Input: part model. Units: mm. Frame: model coordinates. A direction names the side the tool comes from. Round coordinates to 2 decimals unless told otherwise and drop trailing zeros. Write each loop counter-clockwise with the first axis right and the second up, starting at its lowest first coordinate (ties: lowest second). Pieces come first, ordered by that corner, then holes. Notation, with made-up numbers: (60.25, 12.5) -> (80.25, 12.5) arc R11 cw to (80.25, 29.5) -> close; hole circle Ø6 at (-8.75, -35.75). An arc over 180 degrees is marked (long way). Use CSV: the item, a comma, the result in double quotes.
```python
from build123d import *

# Parameters (mm, degrees)
F1_DEPTH = 40
F0_W     = 3
F0_H     = 3
F2_DEPTH = 30
F3_R     = 2
F4_DEPTH = 30
F5_R     = 7.5
F5_R_2   = 5
F6_DEPTH = 5


with BuildPart() as f1:
    # F0 (on Top) → F1 (new body)
    with BuildSketch(Plane.XY):
        with BuildLine():
            ThreePointArc((-4.7696960071, -1.5), (-5, 0), (-4.7696960071, 1.5))
            Line((-4.7696960071, 1.5), (-40, 1.5))
            Line((-40, 1.5), (-40, -1.5))
            Line((-40, -1.5), (-4.7696960071, -1.5))
        make_face()
    extrude(amount=F1_DEPTH)



with BuildPart() as f1b:
    # F0 (on Top) → F1, piece 2 (new body)
    with BuildSketch(Plane.XY):
        with BuildLine():
            ThreePointArc((-1.5, 4.7696960071), (0, 5), (1.5, 4.7696960071))
            Line((1.5, 4.7696960071), (1.5, 40))
            Line((1.5, 40), (-1.5, 40))
            Line((-1.5, 40), (-1.5, 4.7696960071))
        make_face()
    extrude(amount=F1_DEPTH)


with BuildPart() as f1c:
    # F0 (on Top) → F1, piece 3 (new body)
    with BuildSketch(Plane.XY):
        with BuildLine():
            ThreePointArc((4.7696960071, 1.5), (4.9420886291, 0.7587884964), (5, 0))
            ThreePointArc((5, 0), (4.9420886291, -0.7587884964), (4.7696960071, -1.5))
            Line((4.7696960071, -1.5), (40, -1.5))
            Line((40, -1.5), (40, 1.5))
            Line((40, 1.5), (4.7696960071, 1.5))
        make_face()
    extrude(amount=F1_DEPTH)


with BuildPart() as f1d:
    # F0 (on Top) → F1, piece 4 (new body)
    with BuildSketch(Plane.XY):
        with BuildLine():
            Line((1.5, -40), (1.5, -4.7696960071))
            ThreePointArc((1.5, -4.7696960071), (0, -5), (-1.5, -4.7696960071))
            Line((-1.5, -4.7696960071), (-1.5, -40))
            Line((-1.5, -40), (1.5, -40))
        make_face()
    extrude(amount=F1_DEPTH)


with BuildPart() as f1_1:
    add(f1.part)

    add(f1b.part)  # F2 merges F1b

    add(f1c.part)  # F2 merges F1c

    add(f1d.part)  # F2 merges F1d
    # F0 (on Top) → F2 (join)
    with BuildSketch(Plane.XY):
        with BuildLine():
            Line((-1.5, 1.5), (-1.5, 4.7696960071))
            ThreePointArc((-1.5, 4.7696960071), (-3.5355339059, 3.5355339059), (-4.7696960071, 1.5))
            Line((-4.7696960071, 1.5), (-1.5, 1.5))
        make_face()
        with BuildLine():
            Line((1.5, 1.5), (4.7696960071, 1.5))
            ThreePointArc((4.7696960071, 1.5), (3.5355339059, 3.5355339059), (1.5, 4.7696960071))
            Line((1.5, 4.7696960071), (1.5, 1.5))
        make_face()
        with BuildLine():
            ThreePointArc((1.5, -4.7696960071), (3.5355339059, -3.5355339059), (4.7696960071, -1.5))
            Line((4.7696960071, -1.5), (1.5, -1.5))
            Line((1.5, -1.5), (1.5, -4.7696960071))
        make_face()
        with BuildLine():
            ThreePointArc((-4.7696960071, -1.5), (-3.5355339059, -3.5355339059), (-1.5, -4.7696960071))
            Line((-1.5, -4.7696960071), (-1.5, -1.5))
            Line((-1.5, -1.5), (-4.7696960071, -1.5))
        make_face()
        with BuildLine():
            ThreePointArc((4.7696960071, -1.5), (4.9420886291, -0.7587884964), (5, 0))
            ThreePointArc((5, 0), (4.9420886291, 0.7587884964), (4.7696960071, 1.5))
            Line((4.7696960071, 1.5), (1.5, 1.5))
            Line((1.5, 1.5), (1.5, -1.5))
            Line((1.5, -1.5), (4.7696960071, -1.5))
        make_face()
        with BuildLine():
            Line((1.5, 1.5), (1.5, 4.7696960071))
            ThreePointArc((1.5, 4.7696960071), (0, 5), (-1.5, 4.7696960071))
            Line((-1.5, 4.7696960071), (-1.5, 1.5))
            Line((-1.5, 1.5), (1.5, 1.5))
        make_face()
        with BuildLine():
            Line((-1.5, -1.5), (-1.5, 1.5))
            Line((-1.5, 1.5), (-4.7696960071, 1.5))
            ThreePointArc((-4.7696960071, 1.5), (-5, 0), (-4.7696960071, -1.5))
            Line((-4.7696960071, -1.5), (-1.5, -1.5))
        make_face()
        Rectangle(F0_W, F0_H)
        with BuildLine():
            ThreePointArc((-1.5, -4.7696960071), (0, -5), (1.5, -4.7696960071))
            Line((1.5, -4.7696960071), (1.5, -1.5))
            Line((1.5, -1.5), (-1.5, -1.5))
            Line((-1.5, -1.5), (-1.5, -4.7696960071))
        make_face()
    extrude(amount=F2_DEPTH)

    # F3 (on face) → F4 (cut)
    with BuildSketch(Plane.XY.offset(30)):
        Circle(F3_R)
    extrude(amount=-F4_DEPTH, mode=Mode.SUBTRACT)

    # F5 (on face) → F6 (cut)
    with BuildSketch(Plane(origin=(0, 0, 0), x_dir=(1, 0, 0), z_dir=(0, 0, -1))):
        Circle(F5_R)
        Circle(F5_R_2, mode=Mode.SUBTRACT)
    extrude(amount=-F6_DEPTH, mode=Mode.SUBTRACT)


solid = f1_1.part
```
Item 1: Section query A-A on z = 4. Return the cut outline in (x, y).
Worked answers:
outline,"(-40, -1.5) -> (-7.35, -1.5) arc R7.5 cw to (-7.35, 1.5) -> (-40, 1.5) -> close; circle Ø10 at (0, 0); (-1.5, -40) -> (1.5, -40) -> (1.5, -7.35) arc R7.5 cw to (-1.5, -7.35) -> close; (-1.5, 7.35) arc R7.5 cw to (1.5, 7.35) -> (1.5, 40) -> (-1.5, 40) -> close; (7.35, -1.5) -> (40, -1.5) -> (40, 1.5) -> (7.35, 1.5) arc R7.5 cw to start; hole circle Ø4 at (0, 0)"
Item 2: Pull-direction query (Y, two-part tool) for faces 1 (the face through (0, 7.5, 2.5)), 2 (the face through (-22, 1.5, 20)), 3 (the face through (0, -7.5, 2.5)), 4 (the face through (-1.5, -22, 20)); classes: +Y half, -Y half, draft (parallel to the pull), parting line (faces both ways), or undercut.
Worked answers:
face 1,"undercut"
face 2,"+Y half"
face 3,"undercut"
face 4,"draft"
Item 3: First-contact query: pin 1 Ø17.5 at (x, z) = (-17.5, 27.5) entering from +Y; pin 2 Ø10.5 at (x, z) = (-16, 25.5) entering from -Y; pin 3 Ø10.5 at (y, z) = (28, 27.5) entering from -X. Flat tips, straight axial feed; report the tip coordinate or a pass-through.
Worked answers:
pin 1,"stops at y = 1.5"
pin 2,"stops at y = -1.5"
pin 3,"stops at x = -1.5"
Item 4: Set-up query: faces 5 (the face through (1.5, -23, 20)), 6 (the face through (23, 1.5, 20)), 7 (the face through (-5, 0, 35)). Return all of +Z, -Z, +X, -X, +Y, -Y with unobstructed straight access to the full face (end or side cutting, diameter ignored); none if empty.
Worked answers:
face 5,"+Z, -Z, +X, -Y"
face 6,"+Z, -Z, +X, +Y"
face 7,"+Z"
Item 5: Section query B-B on x = 0. Return the cut outline in (y, z), plus the area to 4 significant figures.
Worked answers:
outline,"(-40, 0) -> (-7.5, 0) -> (-7.5, 5) -> (-5, 5) -> (-5, 0) -> (-2, 0) -> (-2, 30) -> (-5, 30) -> (-5, 40) -> (-40, 40) -> close; (2, 0) -> (5, 0) -> (5, 5) -> (7.5, 5) -> (7.5, 0) -> (40, 0) -> (40, 40) -> (5, 40) -> (5, 30) -> (2, 30) -> close"
area,"2,955 mm²"
Item 6: Section query C-C on z = 33. Return the cut outline in (x, y).
Worked answers:
outline,"(-40, -1.5) -> (-4.77, -1.5) arc R5 cw to (-4.77, 1.5) -> (-40, 1.5) -> close; (-1.5, -40) -> (1.5, -40) -> (1.5, -4.77) arc R5 cw to (-1.5, -4.77) -> close; (-1.5, 4.77) arc R5 cw to (1.5, 4.77) -> (1.5, 40) -> (-1.5, 40) -> close; (4.77, -1.5) -> (40, -1.5) -> (40, 1.5) -> (4.77, 1.5) arc R5 cw to start"
Item 7: Section query D-D on z = 20. Return the cut outline in (x, y), plus the area to 3 significant figures.
Worked answers:
outline,"(-40, -1.5) -> (-4.77, -1.5) arc R5 ccw to (-1.5, -4.77) -> (-1.5, -40) -> (1.5, -40) -> (1.5, -4.77) arc R5 ccw to (4.77, -1.5) -> (40, -1.5) -> (40, 1.5) -> (4.77, 1.5) arc R5 ccw to (1.5, 4.77) -> (1.5, 40) -> (-1.5, 40) -> (-1.5, 4.77) arc R5 ccw to (-4.77, 1.5) -> (-40, 1.5) -> close; hole circle Ø4 at (0, 0)"
area,"487 mm²"
Item 8: Line query: line 1 (Y direction, x = 0, z = 7.5); line 2 (X direction, y = 14, z = 17). Output: solid intervals per line, ascending.
Worked answers:
line 1,"y = -40 to -2, 2 to 40"
line 2,"x = -1.5 to 1.5"
